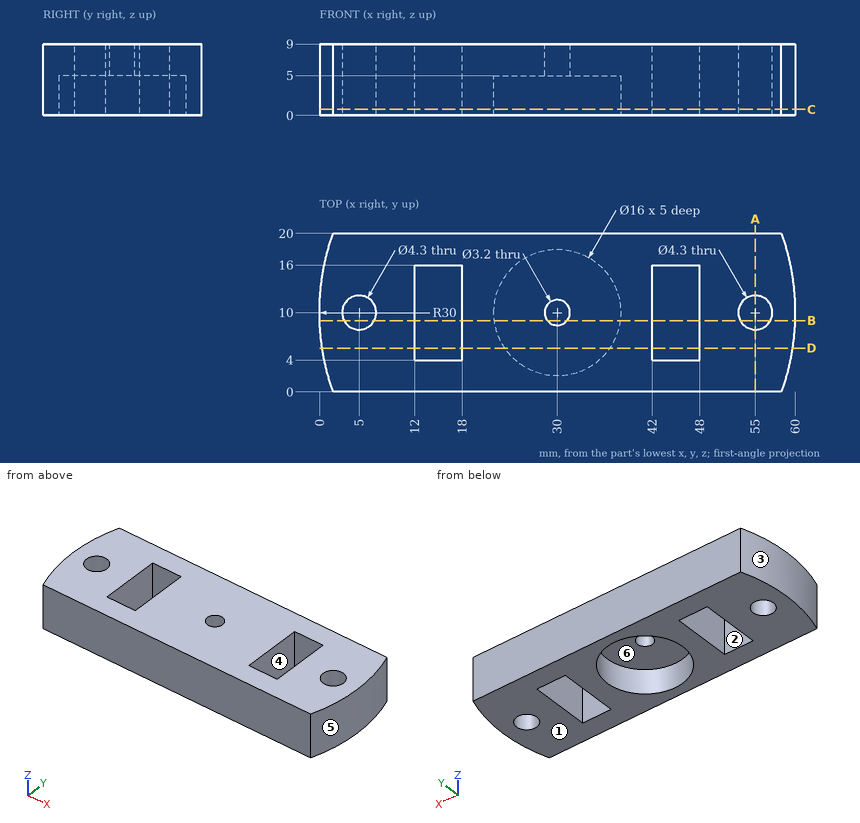
For this review, use the dimensioned drawing (mm, ordinates from the lowest corner) and the shaded views. A direction names the side the tool comes from. Round coordinates to 2 decimals unless told otherwise and drop trailing zeros. Order: outer loops, then holes, each group sorted by start corner. A loop starts at its lowest first (then second) coordinate and runs counter-clockwise, first axis right, second up. Notation, with made-up numbers: (-5.75, 67.5) -> (38.25, 67.5) arc R17 ccw to (38.25, 78.5) -> close; hole circle Ø9 at (-38.5, -31.5). An arc over 180 degrees is marked (long way). One line per item, written item: value. Start each with the question number.
Q1. Take a section at A-A (x = 55). Write out the cut boundary in (y, z).
Q2. Take a section at D-D (y = 5.5). Write out the cut boundary in (x, z).
Q3. Machinability: for the marked faces 4, 5 and 6, which of the approach directions +Z, -Z, +X, -X, +Y, -Y give a long, thin tool a straight path to every point of the face, cutting with its end or side? Answer none if there is none.
Q4. Wall thickness on line 1 (Y direction, x = 5, z = 3.5); line 2 (Y direction, x = 30, z = 2.4); line 3 (X direction, y = 9.75, z = 3): over which ranges is each line inside the solid? List them lowest first.
Q5. Clearance check with flat-ended pins moving along their axes: pin 1 Ø8 at (x, y) = (27, 13.5) entering from -Z; pin 2 Ø1 at (y, z) = (15, 5.5) entering from -X; pin 3 Ø2.5 at (y, z) = (13, 4.5) entering from +X; pin 4 Ø3 at (y, z) = (11, 1) entering from +X. State where each tip first meets the part, or that it passes through.
Q6. Mouldability with a two-part tool opening along X and no side actions: class the marked faces 1, 2 and 3 as released by +X, released by -X, zero draft, split by the parting line, or undercut.
Q7. Take a section at C-C (z = 0.75). Write out the cut boundary in (x, y), and give its area (3 significant figures).
Q8. Take a section at B-B (y = 9). Write out the cut boundary in (x, z).
Reported:
1. outline: (0, 0) -> (7.85, 0) -> (7.85, 9) -> (0, 9) -> close; (12.15, 0) -> (20, 0) -> (20, 9) -> (12.15, 9) -> close
2. outline: (0.34, 0) -> (12, 0) -> (12, 9) -> (0.34, 9) -> close; (18, 0) -> (23.39, 0) -> (23.39, 5) -> (36.61, 5) -> (36.61, 0) -> (42, 0) -> (42, 9) -> (18, 9) -> close; (48, 0) -> (59.66, 0) -> (59.66, 9) -> (48, 9) -> close
3. face 4: +Z, -Z
3. face 5: +Z, -Z, +X
3. face 6: -Z
4. line 1: y = 0 to 7.85, 12.15 to 20
4. line 2: y = 0 to 2, 18 to 20
4. line 3: x = 0 to 2.86, 7.14 to 12, 18 to 22, 38 to 42, 48 to 52.86, 57.14 to 60
5. pin 1: stops at z = 0
5. pin 2: stops at x = 0.34
5. pin 3: stops at x = 59.95
5. pin 4: stops at x = 60
6. face 1: zero draft
6. face 2: undercut
6. face 3: released by -X
7. outline: (1.72, 0) -> (58.28, 0) arc R30 ccw to (58.28, 20) -> (1.72, 20) arc R30 ccw to start; hole circle Ø4.3 at (5, 10); hole (12, 4) -> (18, 4) -> (18, 16) -> (12, 16) -> close; hole circle Ø16 at (30, 10); hole (42, 4) -> (48, 4) -> (48, 16) -> (42, 16) -> close; hole circle Ø4.3 at (55, 10)
7. area: 803 mm2
8. outline: (0.02, 0) -> (3.1, 0) -> (3.1, 9) -> (0.02, 9) -> close; (6.9, 0) -> (12, 0) -> (12, 9) -> (6.9, 9) -> close; (18, 0) -> (22.06, 0) -> (22.06, 5) -> (28.75, 5) -> (28.75, 9) -> (18, 9) -> close; (31.25, 5) -> (37.94, 5) -> (37.94, 0) -> (42, 0) -> (42, 9) -> (31.25, 9) -> close; (48, 0) -> (53.1, 0) -> (53.1, 9) -> (48, 9) -> close; (56.9, 0) -> (59.98, 0) -> (59.98, 9) -> (56.9, 9) -> close
